```python
from build123d import *

# Parameters (mm, degrees)
F1_DEPTH      = 25
F2_R          = 3.175
F3_DEPTH      = 10
F3_DEPTH_BACK = 30.001


with BuildPart() as f1:
    # F0 (on Top) → F1 (new body)
    with BuildSketch(Plane.XY):
        with BuildLine():
            ThreePointArc((12.359207, -8.5), (-15, 0), (12.359207, 8.5))
            Line((12.359207, 8.5), (28.935366, 7.921148))
            ThreePointArc((28.935366, 7.921148), (-30, 0), (28.935366, -7.921148))
            Line((28.935366, -7.921148), (12.359207, -8.5))
        make_face()
    extrude(amount=F1_DEPTH)

    # F2 (on Front) → F3 (cut, two sides)
    with BuildSketch(Plane.XZ) as f3_sk:
        with Locations((-22.5, 12.5)):
            Circle(F2_R)
    extrude(amount=F3_DEPTH, mode=Mode.SUBTRACT)
    extrude(f3_sk.sketch, amount=-F3_DEPTH_BACK, mode=Mode.SUBTRACT)


solid = f1.part
```
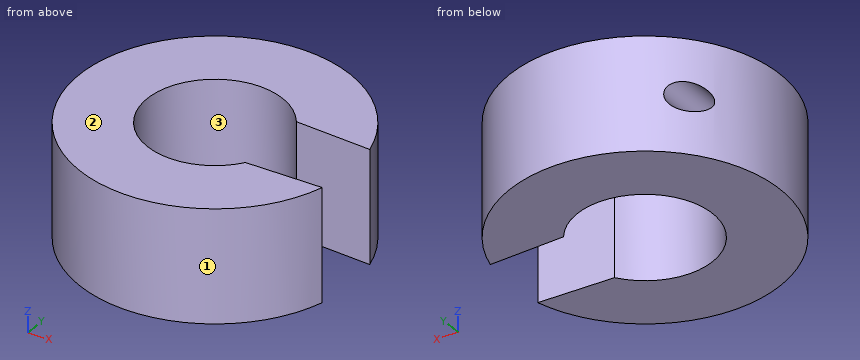
Source: CAD feature listing. Evaluate the final solid. Frame: model axes, mm. Face numbers are marked on the shaded views. Give positions to 0.01 mm unless a question says otherwise; leave off trailing zeros. Write each loop counter-clockwise with the first axis right and the second up, starting at its lowest first coordinate (ties: lowest second). Pieces come first, ordered by that corner, then holes.
1. Pull-direction query (Y, two-part tool) for the marked faces 1, 2 and 3; classes: +Y half, -Y half, draft (parallel to the pull), parting line (faces both ways), or undercut.
2. First-contact query: pin 1 (5 mm diameter, centred on y = -10, z = 20, fed in from +X); pin 2 (8.5 mm diameter, centred on x = -22.5, z = 12.5, fed in from -Y); pin 3 (1 mm diameter, centred on x = 19, z = 6, fed in from -Y). Flat tips, straight axial feed; report the tip coordinate or a pass-through.
3. Section query C-C (y = -1). Return the cut outline in (x, z) (3 decimals).
4. Section query D-D (x = 9.5). Return the cut outline in (y, z).
5. Section query A-A (x = 0). Return the cut outline in (y, z).
6. Section query B-B (y = 10.5). Count the separate pieces of the cut face and the enclosed holes in it, then the cut area to 3 significant figures.
7. Material intervals for line 1 along Y through (x, z) = (0.5, 11.5); line 2 along Z through (x, y) = (-22.5, -1.75) (3 decimals); line 3 along X through (y, z) = (11.5, 12.5) (3 decimals), sorted ascending.
Output values:
1. face 1: parting line
1. face 2: draft
1. face 3: undercut
2. pin 1: stops at x = 28.94
2. pin 2: stops at y = -23.81
2. pin 3: stops at y = -23.62
3. outline: (-29.983, 0) - (-14.967, 0) - (-14.967, 25) - (-29.983, 25) - close; hole circle Ø6.35 at (-22.5, 12.5)
4. outline: (-28.46, 0) - (-11.61, 0) - (-11.61, 25) - (-28.46, 25) - close; (11.61, 0) - (28.46, 0) - (28.46, 25) - (11.61, 25) - close
5. outline: (-30, 0) - (-15, 0) - (-15, 25) - (-30, 25) - close; (15, 0) - (30, 0) - (30, 25) - (15, 25) - close
6. separate pieces: 2
6. enclosed holes: 1
6. area: 838 mm2
7. line 1: y = -30 to -14.99, 14.99 to 30
7. line 2: z = 0 to 9.325, 15.675 to 25
7. line 3: x = -27.708 to -25.675, -19.325 to -9.631, 9.631 to 27.708
